Geometry: final body of the model. Coordinates: model frame, mm. A direction names the side the tool comes from. Coordinates: 2 decimals unless noted, no trailing zeros. Write each loop counter-clockwise with the first axis right and the second up, starting at its lowest first coordinate (ties: lowest second). Pieces come first, ordered by that corner, then holes. Notation, with made-up numbers: (27.5, -3) -> (33.5, -3) arc R22 cw to (33.5, 29) -> close; hole circle Ø8 at (-8, -24.75). An arc over 180 degrees is marked (long way). One line per item, written item: value.
```python
from build123d import *

# Parameters (mm, degrees)
SKETCH2_W           = 152.4
SKETCH2_H           = 195.58
BOSS_EXTRUDE1_DEPTH = 50.8
SHELL1_T            = -5.588


with BuildPart() as part:
    # Sketch2 → Boss-Extrude1 (new body)
    with BuildSketch(Plane(origin=(0, 0, 0), x_dir=(0, 1, 0), z_dir=(0, 0, 1))):
        with Locations((-114.3, 18.147782805)):
            Rectangle(SKETCH2_W, SKETCH2_H)
    extrude(amount=BOSS_EXTRUDE1_DEPTH)

    # Shell1
    shell1_openings = [part.faces().sort_by_distance(p)[0] for p in [
        (-18.147782805, -114.3, 50.8),
        (-115.937782805, -114.3, 25.4),
    ]]
    offset(amount=SHELL1_T, openings=shell1_openings, kind=Kind.INTERSECTION)


solid = part.part
```
(1) Section B-B (z = 46). Return the cut outline in (x, y).
Responses:
outline: (-115.94, -190.5) -> (79.64, -190.5) -> (79.64, -38.1) -> (-115.94, -38.1) -> (-115.94, -43.69) -> (74.05, -43.69) -> (74.05, -184.91) -> (-115.94, -184.91) -> close
(2) First-contact query: pin 1 (22.5 mm diameter, centred on y = -106, z = 37, fed in from -X); pin 2 (8 mm diameter, centred on x = -65.5, y = -149, fed in from +Z). Flat tips, straight axial feed; report the tip coordinate or a pass-through.
Responses:
pin 1: stops at x = 74.05
pin 2: stops at z = 5.59
(3) Pull-direction query (Y, two-part tool) for faces 1 (the flat face through (-17, -38.1, 25)), 2 (the flat face through (-22, -115, 5.588)), 3 (the flat face through (-20, -184.912, 28)), 4 (the flat face through (79.642, -115, 25)); classes: released by +Y, released by -Y, zero draft, split by the parting line, or undercut.
Responses:
face 1: released by +Y
face 2: undercut
face 3: undercut
face 4: zero draft
(4) Line query: line 1 (Y direction, x = -62, z = 32.5); line 2 (Z direction, x = 8, y = -149); line 3 (X direction, y = -97, z = 34). Output: solid intervals per line, ascending. Write a range as [from, to].
Responses:
line 1: y = [-190.5, -184.91], [-43.69, -38.1]
line 2: z = [0, 5.59]
line 3: x = [74.05, 79.64]
(5) Section C-C (y = -172). Return the cut outline in (x, z), then the cut area to 3 significant figures.
Responses:
outline: (-115.94, 0) -> (79.64, 0) -> (79.64, 50.8) -> (74.05, 50.8) -> (74.05, 5.59) -> (-115.94, 5.59) -> close
area: 1,350 mm2
(6) Reachability of faces 5 (the flat face through (74.054, -115, 28)), 6 (the flat face through (-20, -115, 0)) from +Z, -Z, +X, -X, +Y, -Y: full face, straight path, thin tool, end or side. Return the list, or none.
Responses:
face 5: +Z, -X
face 6: -Z, +X, -X, +Y, -Y
(7) Section A-A (x = 7.5). Return the cut outline in (y, z), then the cut area to 3 significant figures.
Responses:
outline: (-190.5, 0) -> (-38.1, 0) -> (-38.1, 50.8) -> (-43.69, 50.8) -> (-43.69, 5.59) -> (-184.91, 5.59) -> (-184.91, 50.8) -> (-190.5, 50.8) -> close
area: 1,360 mm2
